from build123d import *

# Parameters (mm, degrees)
SKETCH1_R           = 1.9
BOSS_EXTRUDE1_DEPTH = 1.65
SKETCH3_W           = 2
SKETCH3_H           = 4.5
BOSS_EXTRUDE2_DEPTH = 0.85
SKETCH4_W           = 6.5
SKETCH4_H           = 5
BOSS_EXTRUDE3_DEPTH = 1.65
SKETCH5_R           = 0.5
CUT_EXTRUDE1_DEPTH  = 17.243306314


with BuildPart() as part:
    # Sketch1 → Boss-Extrude1 (new body)
    with BuildSketch(Plane(origin=(0, 0, 0), x_dir=(1, 0, 0), z_dir=(0, 1, 0))):
        with BuildLine():
            Line((-8.4, -11.25), (8.4, -11.25))
            ThreePointArc((8.4, -11.25), (10.6627417, -10.3127417), (11.6, -8.05))
            Line((11.6, -8.05), (11.6, 8.05))
            ThreePointArc((11.6, 8.05), (10.6627417, 10.3127417), (8.4, 11.25))
            Line((8.4, 11.25), (-8.4, 11.25))
            ThreePointArc((-8.4, 11.25), (-10.6627417, 10.3127417), (-11.6, 8.05))
            Line((-11.6, 8.05), (-11.6, -8.05))
            ThreePointArc((-11.6, -8.05), (-10.6627417, -10.3127417), (-8.4, -11.25))
        make_face()
        with Locations(Location((-8.015151515, 7.773315047, 0), (0, 0, 270))):
            Circle(SKETCH1_R, mode=Mode.SUBTRACT)
        with Locations(Location((8.084848485, 7.909090909, 0), (0, 0, 270))):
            Circle(SKETCH1_R, mode=Mode.SUBTRACT)
        with Locations(Location((8.084848485, -7.840909091, 0), (0, 0, 270))):
            Circle(SKETCH1_R, mode=Mode.SUBTRACT)
        with Locations(Location((-8.015151515, -7.840909091, 0), (0, 0, 270))):
            Circle(SKETCH1_R, mode=Mode.SUBTRACT)
    extrude(amount=BOSS_EXTRUDE1_DEPTH)

    # Sketch3 → Boss-Extrude2 (add)
    with BuildSketch(Plane(origin=(0, 1.65, 0), x_dir=(1, 0, 0), z_dir=(0, 1, 0))):
        with Locations((-3, 7)):
            Rectangle(SKETCH3_W, SKETCH3_H)
        with Locations((0, 7)):
            Rectangle(SKETCH3_W, SKETCH3_H)
        with Locations((3, 7)):
            Rectangle(SKETCH3_W, SKETCH3_H)
        with Locations((3, -7)):
            Rectangle(SKETCH3_W, SKETCH3_H)
        with Locations((0, -7)):
            Rectangle(SKETCH3_W, SKETCH3_H)
        with Locations((-3, -7)):
            Rectangle(SKETCH3_W, SKETCH3_H)
    extrude(amount=BOSS_EXTRUDE2_DEPTH)

    # Sketch4 → Boss-Extrude3 (add)
    with BuildSketch(Plane(origin=(0, 1.65, 0), x_dir=(1, 0, 0), z_dir=(0, 1, 0))):
        Rectangle(SKETCH4_W, SKETCH4_H)
    extrude(amount=BOSS_EXTRUDE3_DEPTH)

    # Sketch5 → Cut-Extrude1 (cut, through all)
    with BuildSketch(Plane(origin=(0, 1.65, 0), x_dir=(1, 0, 0), z_dir=(0, 1, 0))):
        with Locations(Location((-6.615151515, 0, 0), (0, 0, 270))):
            Circle(SKETCH5_R)
        with Locations(Location((-6.615151515, 2.5, 0), (0, 0, 270))):
            Circle(SKETCH5_R)
        with Locations(Location((-6.615151515, -2.5, 0), (0, 0, 270))):
            Circle(SKETCH5_R)
        with Locations(Location((6.684848485, 4.5, 0), (0, 0, 270))):
            Circle(SKETCH5_R)
        with Locations(Location((6.684848485, 2, 0), (0, 0, 270))):
            Circle(SKETCH5_R)
        with Locations(Location((6.684848485, -0.5, 0), (0, 0, 270))):
            Circle(SKETCH5_R)
        with Locations(Location((6.684848485, -3, 0), (0, 0, 270))):
            Circle(SKETCH5_R)
    extrude(amount=-CUT_EXTRUDE1_DEPTH, mode=Mode.SUBTRACT)


solid = part.part
CAD build for the part. Positions are in the model's coordinates, mm. A direction names the side the tool comes from. Coordinates: 2 decimals unless noted, no trailing zeros. Order: outer loops, then holes, each group sorted by start corner. A loop starts at its lowest first (then second) coordinate and runs counter-clockwise, first axis right, second up.
Item 1: Band-saw the part on C-C on y = 0.4. Give the number of separate pieces and of enclosed holes in the cut face, plus the area to 3 significant figures.
Check sheet entries:
separate pieces: 1
enclosed holes: 11
area: 462 mm2
Item 2: Band-saw the part on B-B on z = -1. List the corners of the cut face in (x, y), plus the area to 3 significant figures.
Check sheet entries:
outline: (-11.6, 0) - (11.6, 0) - (11.6, 1.65) - (3.25, 1.65) - (3.25, 3.3) - (-3.25, 3.3) - (-3.25, 1.65) - (-11.6, 1.65) - close
area: 49.0 mm2
Item 3: Band-saw the part on D-D on x = -4.5. List the corners of the cut face in (y, z).
Check sheet entries:
outline: (0, -11.25) - (1.65, -11.25) - (1.65, 11.25) - (0, 11.25) - close
Item 4: Pin check, flat tips, straight feed: pin 1 Ø0.7 at (y, z) = (2.5, -8) entering from +X; pin 2 Ø0.5 at (x, y) = (0.5, 2) entering from +Z; pin 3 Ø2 at (x, z) = (3, -6) entering from +Y. Stop position of each tip, or through.
Check sheet entries:
pin 1: stops at x = 4
pin 2: stops at z = 9.25
pin 3: stops at y = 2.5
Item 5: 3-axis set-ups, long thin cutter, end or side, ignore diameter. For faces 1 (the face through (-3, 2, -4.75)), 2 (the face through (-2, 2, -7)), 3 (the face through (2, 2, 7)), 4 (the face through (3, 2, -9.25)): which of +Z, -Z, +X, -X, +Y, -Y reach the whole face in a straight line?
Check sheet entries:
face 1: +X, -X, +Y
face 2: -Z, +Y
face 3: +Z, +Y
face 4: -Z, +X, -X, +Y
Item 6: Two-plate mould, pull along X, no slides. Class faces 5 (the face through (-3, 2, -9.25)), 6 (the face through (1, 2, -7)), 7 (the face through (-4, 2, 7)): +X half, -X half, draft (parallel to the pull), parting line (faces both ways), or undercut.
Check sheet entries:
face 5: draft
face 6: undercut
face 7: -X half
Item 7: Drill centre lines: L1, parallel to X at y = 2.2, z = 6.5; L2, parallel to Z at x = -7.25, y = 0.6; L3, parallel to Z at x = 9, y = 1.4. Where is each one in solid material? Low to high.
Check sheet entries:
L1: x = -4 to -2, -1 to 1, 2 to 4
L2: z = -11.25 to -9.51, -6.03 to 6.1, 9.58 to 11.25
L3: z = -11.19 to -9.57, -6.24 to 6.18, 9.51 to 11.19
Item 8: Band-saw the part on A-A on z = 8.5. List the corners of the cut face in (x, y).
Check sheet entries:
outline: (-11.57, 0) - (-9.8, 0) - (-9.8, 1.65) - (-11.57, 1.65) - close; (-6.23, 0) - (6.3, 0) - (6.3, 1.65) - (4, 1.65) - (4, 2.5) - (2, 2.5) - (2, 1.65) - (1, 1.65) - (1, 2.5) - (-1, 2.5) - (-1, 1.65) - (-2, 1.65) - (-2, 2.5) - (-4, 2.5) - (-4, 1.65) - (-6.23, 1.65) - close; (9.87, 0) - (11.57, 0) - (11.57, 1.65) - (9.87, 1.65) - close
